Input: dimensioned drawing with shaded views. Units: mm. Origin: part minimum x, y, z. Give positions to 0.01 mm unless a question says otherwise; leave off trailing zeros. Loops run counter-clockwise (first coordinate to the right, second up) from the corner with the lowest first, then second, coordinate; pieces in that order, holes last.
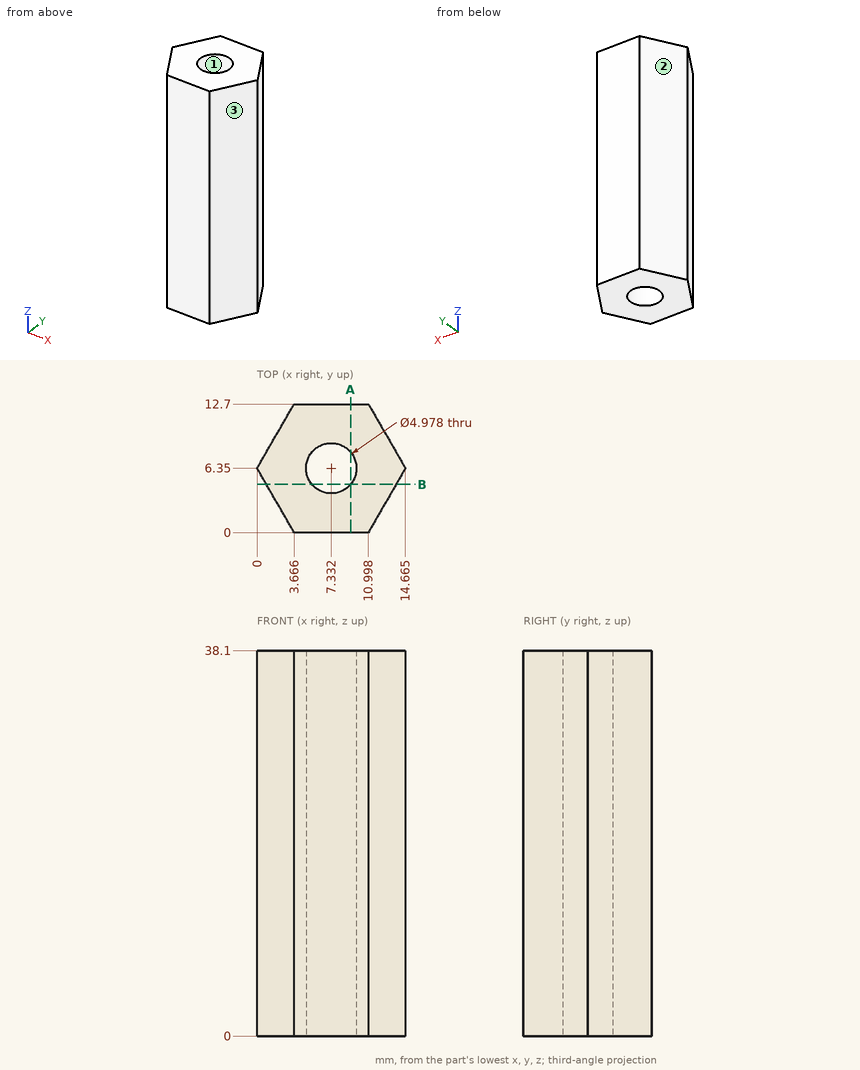
(1) Mould query, pull axis Y, two halves, no side actions, for the marked faces 1, 2 and 3. Classes: pulls with the +Y half, pulls with the -Y half, needs draft (parallel to the pull), parting line crosses it, or undercut.
A:
face 1: undercut
face 2: pulls with the +Y half
face 3: pulls with the -Y half
(2) First-contact query: pin 1 (1.5 mm diameter, centred on y = 5.5, z = 6, fed in from -X). Flat tip, straight axial feed; report the tip coordinate or a pass-through.
A:
pin 1: stops at x = 0.06
(3) Section A-A, the plane x = 9.25. Return the cut outline in (y, z), then the cut area to 3 significant figures.
A:
outline: (0, 0) - (4.76, 0) - (4.76, 38.1) - (0, 38.1) - close; (7.94, 0) - (12.7, 0) - (12.7, 38.1) - (7.94, 38.1) - close
area: 363 mm2
(4) Ray query, line 1 along X through (y, z) = (5.5, 20) (1 decimal); line 2 along X through (y, z) = (6.25, 31) (1 decimal); line 3 along Y through (x, z) = (9, 29.5). Return the intervals inside material, ascending.
A:
line 1: x = 0.5 to 5, 9.7 to 14.2
line 2: x = 0.1 to 4.8, 9.8 to 14.6
line 3: y = 0 to 4.5, 8.2 to 12.7
(5) Section B-B, the plane y = 4.75. Return the cut outline in (x, z) (1 decimal), then the cut area to 3 significant figures.
A:
outline: (0.9, 0) - (5.4, 0) - (5.4, 38.1) - (0.9, 38.1) - close; (9.2, 0) - (13.7, 0) - (13.7, 38.1) - (9.2, 38.1) - close
area: 343 mm2
